from build123d import *

# Parameters (mm, degrees)
BOSS_EXTRUDE1_DEPTH     = 15.875
BOSS_EXTRUDE2_DEPTH     = 11.43
CUT_EXTRUDE1_DEPTH      = 12.43
CUT_EXTRUDE1_DEPTH_BACK = 11.1125


with BuildPart() as part:
    # Sketch1 → Boss-Extrude1 (new body)
    with BuildSketch(Plane.XY):
        with BuildLine():
            Line((0, 0), (36.195, 175.373848891))
            ThreePointArc((36.195, 175.373848891), (104.775, 150.790425527), (173.355, 175.373848891))
            Line((173.355, 175.373848891), (209.55, 0))
            ThreePointArc((209.55, 0), (104.775, -41.729500882), (0, 0))
        make_face()
    extrude(amount=BOSS_EXTRUDE1_DEPTH)

    # Sketch2 → Boss-Extrude2 (add)
    with BuildSketch(Plane.XY):
        Polygon((20.407819149, 98.880999907), (39.064611584, 95.030467992), (37.010994563, 85.080178693), (18.354202128, 88.930710608), align=None)
        Polygon((189.142180851, 98.880999907), (170.485388416, 95.030467992), (172.539005437, 85.080178693), (191.195797872, 88.930710608), align=None)
        with BuildLine():
            Line((121.447738693, -20.993053202), (120.65, -14.693361703))
            Line((120.65, -14.693361703), (88.9, -14.693361703))
            Line((88.9, -14.693361703), (88.102261307, -20.993053202))
            ThreePointArc((88.102261307, -20.993053202), (104.775, -22.044500882), (121.447738693, -20.993053202))
        make_face()
    extrude(amount=-BOSS_EXTRUDE2_DEPTH)

    # Sketch4 → Cut-Extrude1 (cut, two sides)
    with BuildSketch(Plane(origin=(0, 0, 0), x_dir=(-1, 0, 0), z_dir=(0, 0, -1))) as cut_extrude1_sk:
        with BuildLine():
            Line((-174.137297951, 108.751840254), (-181.324957525, 73.925827708))
            Line((-181.324957525, 73.925827708), (-192.270924578, 20.889873244))
            ThreePointArc((-192.270924578, 20.889873244), (-104.775, -14.693361703), (-17.279075422, 20.889873244))
            Line((-17.279075422, 20.889873244), (-28.225042475, 73.925827708))
            Line((-28.225042475, 73.925827708), (-35.412702049, 108.751840254))
            Line((-35.412702049, 108.751840254), (-44.766321163, 154.072469762))
            ThreePointArc((-44.766321163, 154.072469762), (-104.775, 138.090425527), (-164.783678837, 154.072469762))
            Line((-164.783678837, 154.072469762), (-174.137297951, 108.751840254))
        make_face()
    extrude(amount=CUT_EXTRUDE1_DEPTH, mode=Mode.SUBTRACT)
    extrude(cut_extrude1_sk.sketch, amount=-CUT_EXTRUDE1_DEPTH_BACK, mode=Mode.SUBTRACT)


solid = part.part
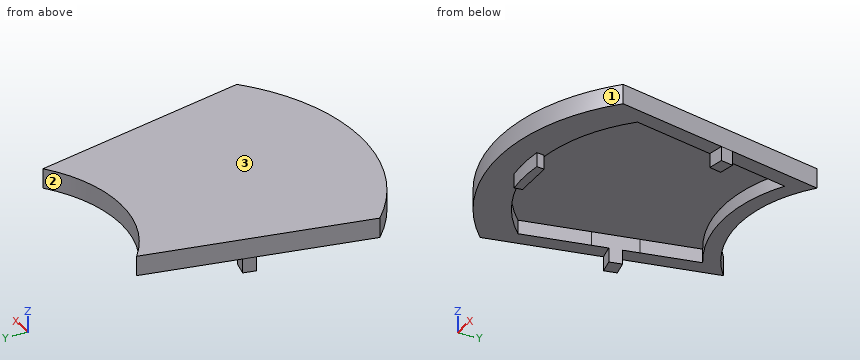
Part model, mm, in its own coordinate system. Face numbers are marked on the shaded views. Give positions to 0.01 mm unless a question says otherwise; leave off trailing zeros. Loops run counter-clockwise (first coordinate to the right, second up) from the corner with the lowest first, then second, coordinate; pieces in that order, holes last. Notation, with made-up numbers: (-9, 71) -> (1, 71) arc R28 cw to (1, 102) -> close; hole circle Ø4 at (39, 15). An arc over 180 degrees is marked (long way). Write each question's results on one line, items separated by ' | '. Start each with the question number.
Q1. Pull direction X, two halves, no side cores. Call the marked faces 1, 2 and 3: +X half, -X half, draft (parallel to the pull), parting line (faces both ways), or undercut.
Q2. Pin check, flat tips, straight feed: P1, Ø4, axis at x = 82, y = 106, coming from the -Z side; P2, Ø1, axis at y = 77.5, z = 6.5, coming from the +X side; P3, Ø12, axis at x = 106, z = 3, coming from the +Y side; P4, Ø6, axis at x = 52.5, z = -4.5, coming from the +Y side. Stop position of each tip, or through.
Q3. Band-saw the part on C-C on x = 159. List the corners of the cut face in (y, z) (1 decimal).
Q4. Band-saw the part on B-B on y = 131. List the corners of the cut face in (x, z) (1 decimal).
Q5. Wall check: L1, parallel to Z at x = 87.5, y = 7 (1 decimal); L2, parallel to X at y = 93, z = 7.75; L3, parallel to Y at x = 81, z = 1.5. Give the ranges that are in metal, low to high.
Results are:
1) face 1: parting line | face 2: undercut | face 3: draft
2) P1: stops at z = 11.11 | P2: stops at x = 193.66 | P3: stops at y = 151.03 | P4: passes through
3) outline: (-31.8, 0) -> (-2.4, 0) -> (-2.4, 11.1) -> (151, 11.1) -> (151, 0) -> (165.4, 0) -> (165.4, 15.9) -> (-31.8, 15.9) -> close
4) outline: (27, 0) -> (40, 0) -> (40, 11.1) -> (169.5, 11.1) -> (169.5, 0) -> (182.5, 0) -> (182.5, 15.9) -> (27, 15.9) -> close
5) L1: z = 11.1 to 15.9 | L2: x = 19.19 to 32.16, 177.39 to 190.36 | L3: y = -39.86 to -12.42, 140.46 to 153.44
